Verification items for the finished model (mm, model axes). Coordinates: 2 decimals unless noted, no trailing zeros. Write each loop counter-clockwise with the first axis right and the second up, starting at its lowest first coordinate (ties: lowest second). Pieces come first, ordered by that corner, then holes. Notation, with made-up numbers: M 55.5,77.25 L 105.5,77.25 A21 ccw 105.5,105.25 Z; hole C 84,-30.5 d2. An arc over 180 degrees is marked long. Answer in a Markdown table with one row per item.
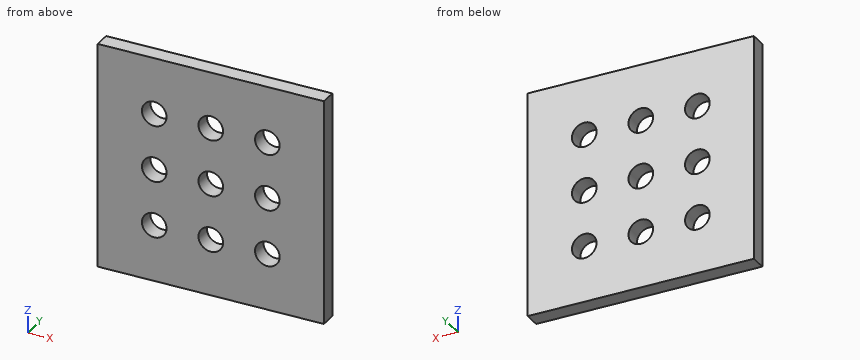
from build123d import *

# Parameters (mm, degrees)
F0_W     = 350
F0_H     = 350
F0_R     = 19.05
F1_DEPTH = 25


with BuildPart() as f1:
    # F0 (on Front) → F1 (new body)
    with BuildSketch(Plane.XZ):
        Rectangle(F0_W, F0_H)
        with Locations((-87.5, -87.5)):
            Circle(F0_R, mode=Mode.SUBTRACT)
        with Locations((0, -87.5)):
            Circle(F0_R, mode=Mode.SUBTRACT)
        with Locations((87.5, -87.5)):
            Circle(F0_R, mode=Mode.SUBTRACT)
        with Locations((-87.5, 0)):
            Circle(F0_R, mode=Mode.SUBTRACT)
        with Locations((-87.5, 87.5)):
            Circle(F0_R, mode=Mode.SUBTRACT)
        Circle(F0_R, mode=Mode.SUBTRACT)
        with Locations((87.5, 0)):
            Circle(F0_R, mode=Mode.SUBTRACT)
        with Locations((0, 87.5)):
            Circle(F0_R, mode=Mode.SUBTRACT)
        with Locations((87.5, 87.5)):
            Circle(F0_R, mode=Mode.SUBTRACT)
    extrude(amount=F1_DEPTH)


solid = f1.part
1) Sectioned sample at C-C (y = -12.5). Give the number of separate pieces and of enclosed holes in the cut face, then the cut area to 3 significant figures.
Response values:
| item | result |
|---|---|
| separate pieces | 1 |
| enclosed holes | 9 |
| area | 112,000 mm² |
2) Thickness scan on L1, parallel to Z at x = 0, y = -7.5; L2, parallel to X at y = -11, z = -88.5; L3, parallel to X at y = -2, z = 6. Record the ranges inside material, lowest first. Write a range as [from, to].
Response values:
| item | result |
|---|---|
| L1 | z = [-175, -106.55], [-68.45, -19.05], [19.05, 68.45], [106.55, 175] |
| L2 | x = [-175, -106.52], [-68.48, -19.02], [19.02, 68.48], [106.52, 175] |
| L3 | x = [-175, -105.58], [-69.42, -18.08], [18.08, 69.42], [105.58, 175] |
3) Sectioned sample at B-B (z = -87.5). Record the cut outline in (x, y).
Response values:
| item | result |
|---|---|
| outline | M -175,-25 L -106.55,-25 L -106.55,0 L -175,0 Z; M -68.45,-25 L -19.05,-25 L -19.05,0 L -68.45,0 Z; M 19.05,-25 L 68.45,-25 L 68.45,0 L 19.05,0 Z; M 106.55,-25 L 175,-25 L 175,0 L 106.55,0 Z |
4) Sectioned sample at A-A (x = 0). Record the cut outline in (y, z).
Response values:
| item | result |
|---|---|
| outline | M -25,-175 L 0,-175 L 0,-106.55 L -25,-106.55 Z; M -25,-68.45 L 0,-68.45 L 0,-19.05 L -25,-19.05 Z; M -25,19.05 L 0,19.05 L 0,68.45 L -25,68.45 Z; M -25,106.55 L 0,106.55 L 0,175 L -25,175 Z |
